Verification items for the finished model (mm, model axes). Give positions to 0.01 mm unless a question says otherwise; leave off trailing zeros. Write each loop counter-clockwise with the first axis right and the second up, starting at its lowest first coordinate (ties: lowest second). Pieces come first, ordered by that corner, then holes. Notation, with made-up numbers: (41.25, 2) -> (72.25, 2) arc R15 cw to (72.25, 30) -> close; hole circle Ø5 at (30, 69.5). An arc over 180 degrees is marked (long way). Use one line per item in the form item = value. Start each with the question number.
(1) Depth check by flat-ended pin: pin 1 Ø2 at (x, z) = (357, 150) entering from -Y; pin 2 Ø8 at (x, y) = (363, 132) entering from -Z; pin 3 Ø1.9 at (x, z) = (3.5, -46.5) entering from +Y; pin 4 Ø3 at (y, z) = (-150, 197) entering from +X. Enter the tip coordinate at first touch or a pass-through.
(2) Scan lines: L1, parallel to X at y = -31.5, z = 126.5; L2, parallel to Z at x = 188, y = -149.5; L3, parallel to X at y = 65, z = 500. Record each from-to range of solid material in increasing order.
(3) Section check A-A, the plane y = 65.5. State how many separate pieces and enclosed holes the cut face has, plus the area to 3 significant figures.
(4) Section check B-B, the plane z = 32.5. Record the cut outline in (x, y), plus the area to 3 significant figures.
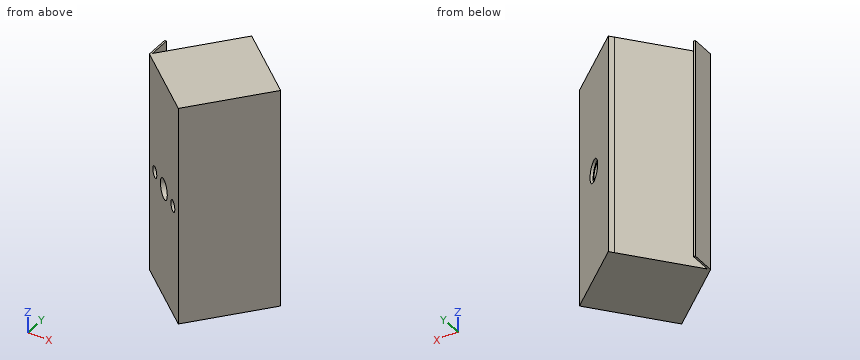
from build123d import *

# Parameters (mm, degrees)
BOSS_EXTRUDE1_DEPTH     = 262.8
CUT_EXTRUDE3_DEPTH      = 560.510929996
CUT_EXTRUDE3_DEPTH_BACK = 560.510929996
SKETCH6_R               = 36
BOSS_EXTRUDE4_DEPTH     = 275
BOSS_EXTRUDE5_DEPTH     = 275
SKETCH11_W              = 305.28
SKETCH11_H              = 812.8
SKETCH11_R              = 31
BOSS_EXTRUDE6_DEPTH     = 10
SKETCH12_W              = 305.28
SKETCH12_H              = 812.8
SKETCH12_R              = 40
BOSS_EXTRUDE7_DEPTH     = 10
SKETCH13_R              = 20.52
CUT_EXTRUDE4_DEPTH      = 170


with BuildPart() as part:
    # Sketch1 → Boss-Extrude1 (new body)
    with BuildSketch(Plane.XY):
        Polygon((0, 0), (0, 86.668071476), (6.393546256, 86.668071476), (6.393546256, 7.619531721), (199.264159003, 237.473777367), (433.122206598, 41.243575882), (233.858047595, -196.230201485), align=None)
    extrude(amount=BOSS_EXTRUDE1_DEPTH)

    # Sketch6 → Cut-Extrude3 (cut, two sides: drawn at the far end of the back side and taken through both)
    with BuildSketch(Plane(origin=(0, 0, 0), x_dir=(-0.7660444431189771, 0.6427876096865406, 0), z_dir=(-0.6427876096865405, -0.766044443118977, 0)).offset(-CUT_EXTRUDE3_DEPTH_BACK)):
        with Locations((-152.64, -131.4)):
            Circle(SKETCH6_R)
    extrude(amount=CUT_EXTRUDE3_DEPTH + CUT_EXTRUDE3_DEPTH_BACK, mode=Mode.SUBTRACT)

    # Sketch7 → Boss-Extrude4 (add)
    with BuildSketch(Plane.XY.offset(262.8)):
        Polygon((233.858047595, -196.230201485), (0, 0), (0, 86.668071476), (6.393546256, 86.668071476), (6.393546256, 7.619531721), (199.264159003, 237.473777367), (433.122206598, 41.243575882), align=None)
    extrude(amount=BOSS_EXTRUDE4_DEPTH)

    # Sketch8 → Boss-Extrude5 (add)
    with BuildSketch(Plane(origin=(0, 0, 0), x_dir=(-1, 0, 0), z_dir=(0, 0, -1))):
        Polygon((0, 0), (0, 86.668071476), (-6.393546256, 86.668071476), (-6.393546256, 7.619531721), (-199.264159003, 237.473777367), (-433.122206598, 41.243575882), (-233.858047595, -196.230201485), align=None)
    extrude(amount=BOSS_EXTRUDE5_DEPTH)

    # Sketch11 → Boss-Extrude6 (add)
    with BuildSketch(Plane(origin=(199.264159003, 237.473777367, 0), x_dir=(0.7660444431189771, -0.6427876096865404, 0), z_dir=(0.6427876096865404, 0.7660444431189771, 0))):
        with Locations((152.64, -131.4)):
            Rectangle(SKETCH11_W, SKETCH11_H)
        with Locations(Location((152.64, -131.4, 0), (0, 0, 180))):
            Circle(SKETCH11_R, mode=Mode.SUBTRACT)
    extrude(amount=BOSS_EXTRUDE6_DEPTH)

    # Sketch12 → Boss-Extrude7 (add)
    with BuildSketch(Plane(origin=(205.6920351, 245.134221798, 0), x_dir=(0.7660444431189771, -0.6427876096865406, 0), z_dir=(0.6427876096865405, 0.766044443118977, 0))):
        with Locations((152.64, -131.4)):
            Rectangle(SKETCH12_W, SKETCH12_H)
        with Locations((152.64, -131.4)):
            Circle(SKETCH12_R, mode=Mode.SUBTRACT)
    extrude(amount=BOSS_EXTRUDE7_DEPTH)

    # Sketch13 → Cut-Extrude4 (cut)
    with BuildSketch(Plane(origin=(0, 0, 0), x_dir=(-0.7660444431189771, 0.6427876096865406, 0), z_dir=(-0.6427876096865405, -0.766044443118977, 0))):
        with Locations(Location((-57.599898279, -131.291749379, 0), (0, 0, 180))):
            Circle(SKETCH13_R)
        with Locations(Location((-247.507544032, -131.291749379, 0), (0, 0, 180))):
            Circle(SKETCH13_R)
    extrude(amount=-CUT_EXTRUDE4_DEPTH, mode=Mode.SUBTRACT)


solid = part.part
Completed:
q1.pin_1 = -50.67
q1.pin_2 = through
q1.pin_3 = 86.67
q1.pin_4 = 273.91
q2.L1 = 74.81 to 126.27, 219.38 to 270.62, 302.01 to 372.08
q2.L2 = -275 to 112.15, 150.43 to 537.8
q2.L3 = 0 to 6.39, 54.54 to 435.92
q3.separate_pieces = 2
q3.enclosed_holes = 2
q3.area = 307,000 mm²
q4.outline = (0, 0) -> (233.86, -196.23) -> (445.98, 56.56) -> (212.12, 252.79) -> (6.39, 7.62) -> (6.39, 86.67) -> (0, 86.67) -> close
q4.area = 101,000 mm²
